CAD build for the part. Positions are in the model's coordinates, mm. Face numbers are marked on the shaded views. A direction names the side the tool comes from. Round coordinates to 2 decimals unless told otherwise and drop trailing zeros. Order: outer loops, then holes, each group sorted by start corner. A loop starts at its lowest first (then second) coordinate and runs counter-clockwise, first axis right, second up. Notation, with made-up numbers: (-17.5, -17) -> (33.5, -17) arc R7 ccw to (33.5, -5) -> close; hole circle Ø11 at (60.25, -29). An arc over 180 degrees is marked (long way). Return JSON: item names as keys, results as strings. Group by question number.
Q1. Which spindle directions (+Z, -Z, +X, -X, +Y, -Y) get a long thin tool onto all of the face, cutting with end or side? Do the marked faces 4, 5 and 6. Say none if no direction does.
Q2. Probe line 1 along Y through (x, z) = (12, -4.5); line 2 along Y through (x, z) = (62, -6.5); line 3 along X through (y, z) = (48, -3.5). List the from-to ranges inside material, lowest first.
Q3. Flat gauge pins, fed straight in: pin 1 (12 mm diameter, centred on y = 10.5, z = -16, fed in from +X); pin 2 (8 mm diameter, centred on x = 32, y = 20.5, fed in from -Z). Where does each tip first touch, or does it go through?
Q4. Cut at D-D (y = 13.5). Write the cut outline in (x, z).
Q5. Mould opens along Y. For the marked faces 1, 2 and 3 say: +Y half, -Y half, draft (parallel to the pull), parting line (faces both ways), or undercut.
Q6. Cut at B-B (y = 26.5). Write the cut outline in (x, z), then the cut area to 3 significant figures.
Q7. Cut at C-C (z = -6). Write the cut outline in (x, y).
Q8. Cut at A-A (x = 12). Write the cut outline in (y, z), then the cut area to 3 significant figures.
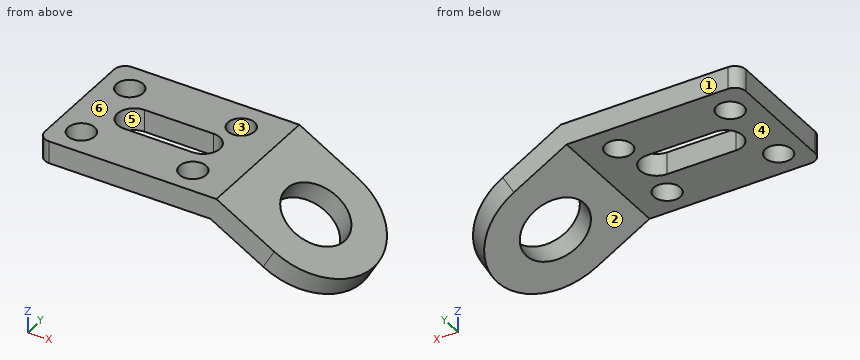
from build123d import *

# Parameters (mm, degrees)
F1_DEPTH = 60
F2_R     = 29.99999
F3_R     = 15
F4_DEPTH = 10
F5_R     = 6
F6_DEPTH = 10
F8_DEPTH = 10
F9_R     = 5


# Not quite as in the source:
# - a fillet or chamfer is up to 0.001 mm smaller than in the source, because OpenCascade refuses the exact size


with BuildPart() as f1:
    # F0 (on Front) → F1 (new body)
    with BuildSketch(Plane.XZ):
        Polygon((80, 0), (0, 0), (0, -10), (77.3205080757, -10), (126.9615242271, -38.6602540378), (131.9615242271, -30), align=None)
    extrude(amount=-F1_DEPTH)

    # F2 (radius 30 in the source; OpenCascade refuses exactly that, so slightly less here)
    f2_edges = [f1.edges().sort_by_distance(p)[0] for p in [
        (129.461524, 0, -34.330127),
        (129.461524, 60, -34.330127),
    ]]
    fillet(f2_edges, radius=F2_R)

    # F3 (on face) → F4 (cut, through all)
    with BuildSketch(Plane(origin=(20, 0, 34.6410161514), x_dir=(0.8660254038, 0, -0.5), z_dir=(0.5, 0, 0.8660254038))):
        with Locations((99.2820323028, 30)):
            Circle(F3_R)
    extrude(amount=-F4_DEPTH, mode=Mode.SUBTRACT)

    # F5 (on face) → F6 (cut, through all)
    with BuildSketch(Plane.XY):
        with Locations((12, 12)):
            Circle(F5_R)
        with Locations((12, 47)):
            Circle(F5_R)
        with Locations((62, 12)):
            Circle(F5_R)
        with Locations((62, 47)):
            Circle(F5_R)
    extrude(amount=-F6_DEPTH, mode=Mode.SUBTRACT)

    # F7 (on face) → F8 (cut, through all)
    with BuildSketch(Plane.XY):
        with BuildLine():
            Line((24.5, 22.5), (55.5, 22.5))
            ThreePointArc((55.5, 22.5), (60.8033008589, 24.6966991411), (63, 30))
            ThreePointArc((63, 30), (60.8033008589, 35.3033008589), (55.5, 37.5))
            Line((55.5, 37.5), (24.5, 37.5))
            ThreePointArc((24.5, 37.5), (19.1966991411, 35.3033008589), (17, 30))
            ThreePointArc((17, 30), (19.1966991411, 24.6966991411), (24.5, 22.5))
        make_face()
    extrude(amount=-F8_DEPTH, mode=Mode.SUBTRACT)

    # F9
    f9_edges = [f1.edges().sort_by_distance(p)[0] for p in [
        (0, 0, -5),
        (0, 60, -5),
    ]]
    fillet(f9_edges, radius=F9_R)


solid = f1.part
Solution:
{
 "1": {"face 4": "-Z, -X, +Y, -Y", "face 5": "+Z, -Z", "face 6": "+Z, +X, -X, +Y, -Y"},
 "2": {"line 1": "y = 0 to 6, 18 to 41, 53 to 60", "line 2": "y = 0 to 6, 18 to 26.26, 33.74 to 41, 53 to 60", "line 3": "x = 0 to 6.08, 17.92 to 56.08, 67.92 to 86.06"},
 "3": {"pin 1": "stops at x = 118.11", "pin 2": "stops at z = -10"},
 "4": {"outline": "(0, -10) -> (6.19, -10) -> (6.19, 0) -> (0, 0) -> close; (17.81, -10) -> (56.19, -10) -> (56.19, 0) -> (17.81, 0) -> close; (67.81, -10) -> (77.32, -10) -> (122.68, -36.19) -> (127.68, -27.53) -> (80, 0) -> (67.81, 0) -> close"},
 "5": {"face 1": "+Y half", "face 2": "draft", "face 3": "undercut"},
 "6": {"outline": "(0, -10) -> (17.87, -10) -> (17.87, 0) -> (0, 0) -> close; (62.13, -10) -> (77.32, -10) -> (88.35, -16.37) -> (93.35, -7.71) -> (80, 0) -> (62.13, 0) -> close; (113.61, -30.95) -> (126.78, -38.56) -> (131.78, -29.9) -> (118.61, -22.29) -> close", "area": "637 mm²"},
 "7": {"outline": "(0, 5) arc R5 ccw to (5, 0) -> (90.39, 0) -> (90.39, 60) -> (5, 60) arc R5 ccw to (0, 55) -> close; hole circle Ø12 at (12, 12); hole circle Ø12 at (12, 47); hole (24.5, 22.5) -> (55.5, 22.5) arc R7.5 ccw to (55.5, 37.5) -> (24.5, 37.5) arc R7.5 ccw to start; hole circle Ø12 at (62, 12); hole circle Ø12 at (62, 47)"},
 "8": {"outline": "(0, -10) -> (6, -10) -> (6, 0) -> (0, 0) -> close; (18, -10) -> (41, -10) -> (41, 0) -> (18, 0) -> close; (53, -10) -> (60, -10) -> (60, 0) -> (53, 0) -> close", "area": "360 mm²"}
}
